Build history of the part. All positions in model axes, mm. A direction names the side the tool comes from. Round coordinates to 2 decimals unless told otherwise and drop trailing zeros. Loops run counter-clockwise (first coordinate to the right, second up) from the corner with the lowest first, then second, coordinate; pieces in that order, holes last. Notation, with made-up numbers: (7, 8.25) -> (30, 8.25) arc R9 cw to (30, 18.25) -> close; hole circle Ø6 at (-17, 43.25). An arc over 180 degrees is marked (long way). Put each result on its own line as item: value. Start each with the question number.
Item 1: Cut at B-B, the plane y = 7.25. List the corners of the cut face in (x, z).
Item 2: Tool access for faces 1 (the flat face through (25, 3, -18)), 2 (the flat face through (0, 0, 0)), 3 (the flat face through (23, 10, -16)): list every direction of +Z, -Z, +X, -X, +Y, -Y with a clear straight run to the whole face (end or side of a thin tool).
Item 3: Cut at C-C, the plane z = 0. List the corners of the cut face in (x, y).
Item 4: Drill centre lines: probe 1 along Z at (x, y) = (11.9, -1.75); probe 2 along Y at (x, z) = (29.5, -17.15); probe 3 along Y at (x, z) = (8.5, 1.75). Where is each one in solid material? Low to high. Write a range as [from, to].
Item 5: Pull direction Z, two halves, no side cores. Call faces 4 (the flat face through (0, -1, -5)), 5 (the cylindrical face through (10.25, -1.48, 0.07)), 6 (the cylindrical face through (-13.55, -1.48, 0.07)), 7 (the flat face through (17.5, 5, -13)): +Z half, -Z half, draft (parallel to the pull), parting line (faces both ways), or undercut.
Item 6: Flat gauge pins, fed straight in: pin 1 Ø6 at (x, z) = (0, 1) entering from +Y; pin 2 Ø4 at (x, z) = (11.9, 0) entering from -Y; pin 3 Ø0.9 at (x, y) = (1.5, -1) entering from -Z; pin 4 Ø0.9 at (x, z) = (25, -17) entering from -Y. Where does each tip first touch, or does it go through?
Item 7: Cut at A-A, the plane x = 11.9. List the corners of the cut face in (y, z), plus the area to 3 significant figures.
Item 8: Cut at D-D, the plane x = 24.5. List the corners of the cut face in (y, z).
```python
from build123d import *

# Parameters (mm, degrees)
F0_W     = 35
F0_H     = 10
F0_R     = 1.65
F1_DEPTH = 3
F2_W     = 24
F2_H     = 24
F3_DEPTH = 3
F4_R     = 6.25
F5_DEPTH = 3
F6_R     = 21
F7_DEPTH = 3


with BuildPart() as f1:
    # F0 (on Front) → F1 (new body)
    with BuildSketch(Plane.XZ):
        Rectangle(F0_W, F0_H)
        with Locations((-11.9, 0)):
            Circle(F0_R, mode=Mode.SUBTRACT)
        with Locations((11.9, 0)):
            Circle(F0_R, mode=Mode.SUBTRACT)
    extrude(amount=F1_DEPTH)

    # F2 (on face) → F3 (join)
    with BuildSketch(Plane.YZ.offset(17.5)):
        with Locations((9, -7)):
            Rectangle(F2_W, F2_H)
    extrude(amount=F3_DEPTH)

    # F4 (on face) → F5 (join)
    with BuildSketch(Plane(origin=(0, 0, -19), x_dir=(1, 0, 0), z_dir=(0, 0, -1))):
        with BuildLine():
            Line((20.5, -21), (29.5, -21))
            ThreePointArc((29.5, -21), (38.5, -12), (29.5, -3))
            Line((29.5, -3), (20.5, -3))
            Line((20.5, -3), (20.5, -21))
        make_face()
        with Locations((29.5, -12)):
            Circle(F4_R, mode=Mode.SUBTRACT)
    extrude(amount=-F5_DEPTH)

    # F6 (on face) → F7 (cut)
    with BuildSketch(Plane.YZ.offset(20.5)):
        with Locations((21, 5)):
            Circle(F6_R)
    extrude(amount=-F7_DEPTH, mode=Mode.SUBTRACT)


solid = f1.part
```
Reply:
1. outline: (17.5, -19) -> (25.44, -19) -> (25.44, -16) -> (20.5, -16) -> (20.5, -10.87) -> (17.5, -10.87) -> close; (33.56, -19) -> (37.14, -19) -> (37.14, -16) -> (33.56, -16) -> close
2. face 1: +Z, -Z, +X, -Y
2. face 2: +Z, -Z, -X, +Y
2. face 3: +Z, +X, +Y, -Y
3. outline: (-17.5, -3) -> (-13.55, -3) -> (-13.55, 0) -> (-17.5, 0) -> close; (-10.25, -3) -> (10.25, -3) -> (10.25, 0) -> (-10.25, 0) -> close; (13.55, -3) -> (20.5, -3) -> (20.5, 0.6) -> (17.5, 0.6) -> (17.5, 0) -> (13.55, 0) -> close
4. probe 1: z = [-5, -1.65], [1.65, 5]
4. probe 2: y = [3, 5.75], [18.25, 21]
4. probe 3: y = [-3, 0]
5. face 4: -Z half
5. face 5: undercut
5. face 6: undercut
5. face 7: draft
6. pin 1: stops at y = 0
6. pin 2: stops at y = -3
6. pin 3: stops at z = -5
6. pin 4: stops at y = 3
7. outline: (-3, -5) -> (0, -5) -> (0, -1.65) -> (-3, -1.65) -> close; (-3, 1.65) -> (0, 1.65) -> (0, 5) -> (-3, 5) -> close
7. area: 20.1 mm^2
8. outline: (3, -19) -> (8.25, -19) -> (8.25, -16) -> (3, -16) -> close; (15.75, -19) -> (21, -19) -> (21, -16) -> (15.75, -16) -> close
